Geometry check sheet. Reference: drawing and pictorial views, mm from the part's lowest x, y, z. A direction names the side the tool comes from. Round coordinates to 2 decimals unless told otherwise and drop trailing zeros. Write each loop counter-clockwise with the first axis right and the second up, starting at its lowest first coordinate (ties: lowest second). Pieces come first, ordered by that corner, then holes. Notation, with made-up numbers: (-31, -24.75) -> (11, -24.75) arc R6 ccw to (11, -20.75) -> close; hole circle Ø1 at (41.5, 58.25). An arc over 180 degrees is marked (long way). Answer as a JSON object with one key per item and string values. Group by question number.
(1) Set-up check for the marked faces 5 and 6: record each of +Z, -Z, +X, -X, +Y, -Y from which the full face is reachable in a straight line by a thin tool's end or side.
(2) Scan lines: L1, parallel to X at y = 30, z = 21.5; L2, parallel to Y at x = 8, z = 12.5; L3, parallel to Z at x = 29.5, y = 14. Record each from-to range of solid material in increasing order. Write a range as from..to.
(3) Sectioned sample at C-C on x = 49. Record the cut outline in (y, z).
(4) Sectioned sample at B-B on y = 15. Record the cut outline in (x, z).
(5) Gauge pin test, flat end, axial feed: pin 1 Ø10.5 at (x, y) = (25.5, 14) entering from -Z. Record the tip position at first contact, or that the pin passes through.
(6) Sectioned sample at A-A on z = 14.5. Record the cut outline in (x, y) (1 decimal).
(7) Draft check along Y on the marked faces 1, 2, 3 and 4. Enter one of: released by +Y, released by -Y, zero draft, split by the parting line, or undercut.
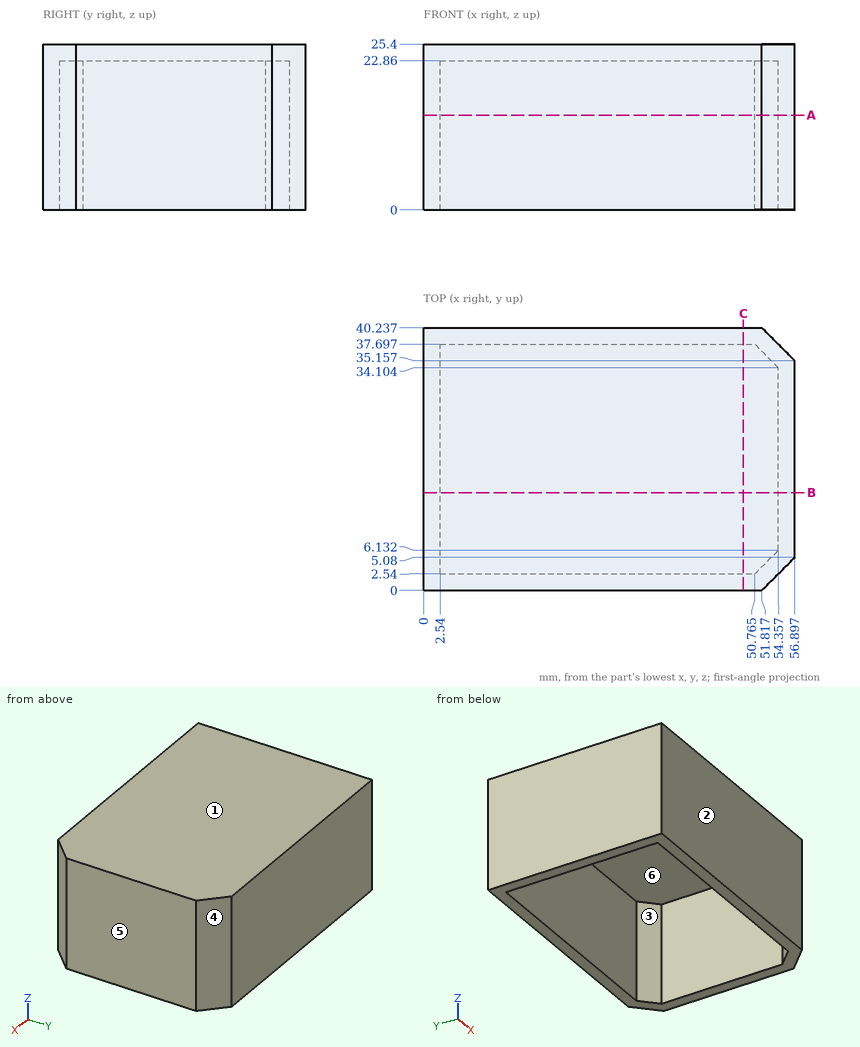
Computed values:
{
 "1": {"face 5": "+Z, -Z, +X, +Y, -Y", "face 6": "-Z"},
 "2": {"L1": "0..2.54, 54.36..56.9", "L2": "0..2.54, 37.7..40.24", "L3": "22.86..25.4"},
 "3": {"outline": "(0, 0) -> (2.54, 0) -> (2.54, 22.86) -> (37.7, 22.86) -> (37.7, 0) -> (40.24, 0) -> (40.24, 25.4) -> (0, 25.4) -> close"},
 "4": {"outline": "(0, 0) -> (2.54, 0) -> (2.54, 22.86) -> (54.36, 22.86) -> (54.36, 0) -> (56.9, 0) -> (56.9, 25.4) -> (0, 25.4) -> close"},
 "5": {"pin 1": "z = 22.86"},
 "6": {"outline": "(0, 0) -> (51.8, 0) -> (56.9, 5.1) -> (56.9, 35.2) -> (51.8, 40.2) -> (0, 40.2) -> close; hole (2.5, 2.5) -> (50.8, 2.5) -> (54.4, 6.1) -> (54.4, 34.1) -> (50.8, 37.7) -> (2.5, 37.7) -> close"},
 "7": {"face 1": "zero draft", "face 2": "released by -Y", "face 3": "undercut", "face 4": "released by +Y"}
}
